Verification items for the finished model (mm, model axes). A direction names the side the tool comes from. Round coordinates to 2 decimals unless told otherwise and drop trailing zeros. Order: outer loops, then holes, each group sorted by start corner. A loop starts at its lowest first (then second) coordinate and runs counter-clockwise, first axis right, second up. Notation, with made-up numbers: M -8.5,39 L 40.5,39 A31 cw 40.5,75 Z; hole C 62,67 d9. An arc over 180 degrees is marked long. Use one line per item in the form item = value. Start each with the question number.
Item 1: Cross-section at C-C on x = 11.5. Enter the section's corners in (y, z).
Item 2: Cross-section at D-D on y = 5. Enter the section's corners in (x, z).
Item 3: Cross-section at B-B on y = 1.5. Enter the section's corners in (x, z).
Item 4: Thickness scan on probe 1 along X at (y, z) = (1.75, -11.25); probe 2 along X at (y, z) = (1.5, -19.5); probe 3 along Z at (x, y) = (20, 1.75). Record the ranges inside material, lowest first. Write a range as [from, to].
Item 5: Go/stop test with flat-tipped pins: pin 1 Ø8 at (x, z) = (15, -10.5) entering from +Y; pin 2 Ø0.8 at (y, z) = (8.5, -8) entering from -X; pin 3 Ø4 at (x, y) = (12, 3.5) entering from +Z; pin 4 Ø2.5 at (y, z) = (2.5, -9) entering from -X. Record where each tip stops, or that it passes through.
Item 6: Release check for a two-part mould opening along Z. For faces 6 (the flat face through (0, 0.4, -11.8)), 7 (the flat face through (19, 4, -24)), 8 (the flat face through (2, 8.5, -9.5)) record: +Z half, -Z half, draft (parallel to the pull), parting line (faces both ways), or undercut.
Item 7: Cross-section at A-A on z = -11.5. Enter the section's corners in (x, y), then the cut area to 3 significant figures.
Item 8: Tool access check on faces 1 (the flat face through (1, 8.5, -16)), 2 (the flat face through (2, 8, -12)), 3 (the flat face through (6, 1, -12)), 4 (the flat face through (18.38, 2, -12)), 5 (the flat face through (3, 8.5, -12.1)). Record the directions out of +Z, -Z, +X, -X, +Y, -Y that give a thin tool (end or side, any length) a straight path to the whole face; none if there is none.
from build123d import *

# Parameters (mm, degrees)
SKETCH1_W           = 40
SKETCH1_H           = 24
BOSS_EXTRUDE1_DEPTH = 1
SKETCH2_W           = 40
SKETCH2_H           = 24
SKETCH2_W_2         = 21
SKETCH2_H_2         = 17.5
SKETCH2_W_3         = 13
SKETCH2_H_3         = 18
BOSS_EXTRUDE3_DEPTH = 8
SKETCH3_W           = 1
SKETCH3_H           = 17.5
CUT_EXTRUDE2_DEPTH  = 3
SKETCH4_W           = 10.24
SKETCH4_H           = 11.92
BOSS_EXTRUDE4_DEPTH = 1.21
CUT_EXTRUDE3_DEPTH  = 2
SKETCH8_W           = 4
SKETCH8_H           = 18
CUT_EXTRUDE4_DEPTH  = 5
SKETCH11_W          = 24
SKETCH11_H          = 9
CUT_EXTRUDE5_DEPTH  = 2
SKETCH12_W          = 4
SKETCH12_H          = 3
CUT_EXTRUDE6_DEPTH  = 3
BOSS_EXTRUDE5_DEPTH = 1


with BuildPart() as part:
    # Sketch1 → Boss-Extrude1 (new body)
    with BuildSketch(Plane(origin=(0, 0, 0), x_dir=(1, 0, 0), z_dir=(0, 1, 0))):
        with Locations((20, 12)):
            Rectangle(SKETCH1_W, SKETCH1_H)
    extrude(amount=BOSS_EXTRUDE1_DEPTH)

    # Sketch2 → Boss-Extrude3 (add)
    with BuildSketch(Plane(origin=(0, 1, 0), x_dir=(1, 0, 0), z_dir=(0, 1, 0))):
        with Locations((20, 12)):
            Rectangle(SKETCH2_W, SKETCH2_H)
        with Locations((11.5, 12)):
            Rectangle(SKETCH2_W_2, SKETCH2_H_2, mode=Mode.SUBTRACT)
        with Locations((29.5, 12)):
            Rectangle(SKETCH2_W_3, SKETCH2_H_3, mode=Mode.SUBTRACT)
    extrude(amount=BOSS_EXTRUDE3_DEPTH)

    # Sketch3 → Cut-Extrude2 (cut)
    with BuildSketch(Plane(origin=(0, 9, 0), x_dir=(1, 0, 0), z_dir=(0, 1, 0))):
        with Locations((22.5, 12)):
            Rectangle(SKETCH3_W, SKETCH3_H)
    extrude(amount=-CUT_EXTRUDE2_DEPTH, mode=Mode.SUBTRACT)

    # Sketch4 → Boss-Extrude4 (add)
    with BuildSketch(Plane(origin=(0, 1, 0), x_dir=(1, 0, 0), z_dir=(0, 1, 0))):
        with Locations((13.26, 12)):
            Rectangle(SKETCH4_W, SKETCH4_H)
    extrude(amount=BOSS_EXTRUDE4_DEPTH)

    # Sketch5 → Cut-Extrude3 (cut)
    with BuildSketch(Plane(origin=(1, 0, 0), x_dir=(0, 0, -1), z_dir=(1, 0, 0))):
        with BuildLine():
            Line((7.53, 2.25), (7.53, 2.96))
            Line((7.53, 2.96), (7.53, 9))
            Line((7.53, 9), (16.47, 9))
            Line((16.47, 9), (16.47, 2.96))
            Line((16.47, 2.96), (16.47, 2.25))
            ThreePointArc((16.47, 2.25), (16.103883476, 1.366116524), (15.22, 1))
            Line((15.22, 1), (8.78, 1))
            ThreePointArc((8.78, 1), (7.896116524, 1.366116524), (7.53, 2.25))
        make_face()
    extrude(amount=-CUT_EXTRUDE3_DEPTH, mode=Mode.SUBTRACT)

    # Sketch8 → Cut-Extrude4 (cut)
    with BuildSketch(Plane(origin=(0, 9, 0), x_dir=(1, 0, 0), z_dir=(0, 1, 0))):
        with Locations((38, 12)):
            Rectangle(SKETCH8_W, SKETCH8_H)
    extrude(amount=-CUT_EXTRUDE4_DEPTH, mode=Mode.SUBTRACT)

    # Sketch11 → Cut-Extrude5 (cut)
    with BuildSketch(Plane(origin=(40, 0, 0), x_dir=(0, 0, -1), z_dir=(1, 0, 0))):
        with Locations((12, 4.5)):
            Rectangle(SKETCH11_W, SKETCH11_H)
    extrude(amount=-CUT_EXTRUDE5_DEPTH, mode=Mode.SUBTRACT)

    # Sketch12 → Cut-Extrude6 (cut)
    with BuildSketch(Plane(origin=(0, 9, 0), x_dir=(1, 0, 0), z_dir=(0, 1, 0))):
        with Locations((6, 2.5)):
            Rectangle(SKETCH12_W, SKETCH12_H)
    extrude(amount=-CUT_EXTRUDE6_DEPTH, mode=Mode.SUBTRACT)

    # Sketch13 → Boss-Extrude5 (add)
    with BuildSketch(Plane(origin=(0, 9, 0), x_dir=(1, 0, 0), z_dir=(0, 1, 0))):
        Polygon((1, 20.75), (3, 20.75), (3, 3.25), (1, 3.25), (1, 7.53), (1, 8.5), (2, 8.5), (2, 10.5), (1, 10.5), (1, 13.5), (2, 13.5), (2, 15.5), (1, 15.5), (1, 16.47), align=None)
    extrude(amount=-BOSS_EXTRUDE5_DEPTH)


solid = part.part
Output values:
q1.outline = M 0,-24 L 9,-24 L 9,-20.75 L 1,-20.75 L 1,-17.96 L 2.21,-17.96 L 2.21,-6.04 L 1,-6.04 L 1,-3.25 L 9,-3.25 L 9,0 L 0,0 Z
q2.outline = M 0,-24 L 38,-24 L 38,-21 L 23,-21 L 23,-3 L 38,-3 L 38,0 L 0,0 L 0,-7.53 L 1,-7.53 L 1,-3.25 L 22,-3.25 L 22,-20.75 L 1,-20.75 L 1,-16.47 L 0,-16.47 Z
q3.outline = M 0,-24 L 38,-24 L 38,0 L 0,0 L 0,-7.78 L 1,-7.78 L 1,-3.25 L 22,-3.25 L 22,-20.75 L 1,-20.75 L 1,-16.22 L 0,-16.22 Z; M 8.14,-17.96 L 18.38,-17.96 L 18.38,-6.04 L 8.14,-6.04 Z; hole M 23,-21 L 36,-21 L 36,-3 L 23,-3 Z
q4.probe_1 = [8.14, 18.38], [22, 23], [36, 38]
q4.probe_2 = [0, 1], [22, 23], [36, 38]
q4.probe_3 = [-24, -20.75], [-3.25, 0]
q5.pin_1 = 2.21
q5.pin_2 = 1
q5.pin_3 = 0
q5.pin_4 = 8.14
q6.face_6 = draft
q6.face_7 = -Z half
q6.face_8 = undercut
q7.outline = M 0,0 L 38,0 L 38,4 L 36,4 L 36,1 L 23,1 L 23,6 L 22,6 L 22,1 L 18.38,1 L 18.38,2.21 L 8.14,2.21 L 8.14,1 L 0,1 Z; M 1,8 L 3,8 L 3,9 L 1,9 Z
q7.area = 63.4 mm2
q8.face_1 = -X, +Y
q8.face_2 = +X
q8.face_3 = none
q8.face_4 = +Y
q8.face_5 = +X, +Y
